Autodesk Inventor part; units mm, degrees
ref_plane "YZ Plane" through (0, 0, 0) normal (1, 0, 0) x (0, 1, 0)
ref_plane "XZ Plane" through (0, 0, 0) normal (0, 1, 0) x (-1, 0, 0)
ref_plane "XY Plane" through (0, 0, 0) normal (0, 0, 1) x (1, 0, 0)
ref_plane "Work Plane1" through (0, 0, 0) normal (0, 0, 1) x (1, 0, 0)
sketch "Sketch1" plane through (0, 0, 0) normal (0, 0, 1) x (1, 0, 0)
  line L0 (96.063, 0.903) -> (102.063, 0.903)
  line L1 (102.063, 0.903) -> (102.063, 3.903)
  line L2 (102.063, 3.903) -> (96.063, 3.903)
  line L3 (96.063, 3.903) -> (96.063, 0.903)
  line L4 (96.063, 0.903) -> (102.063, 3.903) construction
  line L5 (102.063, 0.903) -> (96.063, 3.903) construction
  line L6 (117.163, 0.353) -> (117.163, 4.453)
  line L7 (123.363, 4.453) -> (123.363, 0.353)
  line L8 (117.163, 2.403) -> (123.363, 2.403)
  line L9 (117.263, 3.903) -> (123.263, 3.903)
  line L10 (123.263, 3.903) -> (123.263, 0.903)
  line L11 (123.263, 0.903) -> (117.263, 0.903)
  line L12 (117.263, 0.903) -> (117.263, 3.903)
  line L13 (117.263, 3.903) -> (123.263, 0.903) construction
  line L14 (123.263, 3.903) -> (117.263, 0.903) construction
  point P0 (0, 0)
  point P1 (99.063, 2.403)
  point P2 (120.263, 2.403)
  dimension "d0" = 6
  dimension "d1" = 3
  dimension "d2" = 6
  dimension "d3" = 3
extrude "Extrusion1" add sketch "Sketch1" against normal blind 3
sketch "Sketch2" plane through (0, 0, 0) normal (0, 0, 1) x (1, 0, 0)
  line L0 (96.063, 0.903) -> (102.063, 0.903)
  line L1 (102.063, 0.903) -> (102.063, 3.903)
  line L2 (102.063, 3.903) -> (96.063, 3.903)
  line L3 (96.063, 3.903) -> (96.063, 0.903)
  line L4 (117.263, 3.903) -> (123.263, 3.903)
  line L5 (117.263, 0.903) -> (117.263, 3.903)
  line L6 (123.263, 0.903) -> (117.263, 0.903)
  line L7 (123.263, 3.903) -> (123.263, 0.903)
  point P0 (0, 0)
sketch "Sketch3" plane through (0, 0, 0) normal (0, 0, 1) x (1, 0, 0)
  line L0 (89.663, 3.903) -> (129.663, 3.903)
  line L1 (129.663, 3.903) -> (129.663, 0.903)
  line L2 (129.663, 0.903) -> (89.663, 0.903)
  line L3 (89.663, 0.903) -> (89.663, 3.903)
  line L4 (89.663, 3.903) -> (129.663, 0.903) construction
  line L5 (129.663, 3.903) -> (89.663, 0.903) construction
  point P0 (0, 0)
  point P1 (109.663, 2.403)
  dimension "d6" = 40
  dimension "d7" = 3
extrude "Extrusion2" add sketch "Sketch3" along normal blind 60
sketch "Sketch4" plane through (96.063, 3.903, -3) normal (0, 1, 0) x (1, 0, 0)
  line L0 (-6.4, -63) -> (33.6, -63)
  line L1 (33.6, -3) -> (33.6, -63)
  line L2 (-6.4, -63) -> (33.6, -63)
  line L3 (33.6, -63) -> (33.6, -23)
  line L4 (33.6, -23) -> (-6.4, -23)
  line L5 (-6.4, -23) -> (-6.4, -63)
  circle A0 centre (13.6, -43) radius 19
  line L6 (13.6, -43) -> (13.6, -27)
  line L7 (13.6, -27) -> (-2.4, -27)
  circle A1 centre (-2.4, -27) radius 1.6
  circle A2 centre (29.6, -27) radius 1.6
  line L8 (13.6, -43) -> (17.3038, -43)
  circle A3 centre (-2.4, -59) radius 1.6
  circle A4 centre (29.6, -59) radius 1.6
  point P0 (-96.063, -3)
  dimension "d10" = 40
  dimension "d11" = 38
  dimension "d12" = 16
  dimension "d13" = 16
  dimension "d14" = 3.2
extrude "Extrusion3" cut sketch "Sketch4" against normal through all contours A0 | A1 | A2 | A3 | A4
fillet "Fillet1" radius 2 2 edges at (89.663, 2.403, 60) (129.663, 2.403, 60)
sketch "Sketch5" plane through (117.263, 3.903, -3) normal (0, 1, 0) x (1, 0, 0)
  line L0 (-41.845, -71.0861) -> (34.1344, -71.0861)
  line L1 (34.1344, -71.0861) -> (34.1344, -32.9739)
  line L2 (34.1344, -32.9739) -> (-41.845, -32.9739)
  line L3 (-41.845, -32.9739) -> (-41.845, -71.0861)
  point P0 (-117.263, -3)
extrude "Extrusion4" cut sketch "Sketch5" against normal blind 40
fillet "Fillet2" radius 2 4 edges at (125.8023, 2.403, 29.9739) (93.5237, 2.403, 29.9739) (129.663, 2.403, 29.9739) (89.663, 2.403, 29.9739)
sketch "Sketch6" plane through (117.263, 3.903, -3) normal (0, 1, 0) x (1, 0, 0)
  line L0 (-9.2, 0) -> (-9.2, -3)
  line L1 (-6, 0) -> (-6, -3)
  line L2 (38.3326, -3) -> (-143.1956, -3)
  line L3 (0, -3) -> (-15.2, -3)
  line L4 (-7.6, -3) -> (-6.1, -3)
  line L5 (-6.1, -13.7) -> (-7.6, -13.7)
  line L6 (-7.6, -3) -> (-9.1, -3)
  line L7 (-9.1, -13.7) -> (-7.6, -13.7)
  line L8 (-9.1, -3) -> (-9.1, -9)
  line L9 (-9.1, -9) -> (-10.3, -9)
  line L10 (-10.3, -9) -> (-10.3, -11)
  line L11 (-10.3, -11) -> (-9.1, -11)
  line L12 (-9.1, -3) -> (-9.1, -9)
  line L13 (-9.1, -11) -> (-9.1, -13.7)
  line L14 (-7.6, -3) -> (-7.6, -5.4805)
  line L15 (-6.1, -3) -> (-6.1, -9)
  line L16 (-6.1, -9) -> (-4.9, -9)
  line L17 (-4.9, -9) -> (-4.9, -11)
  line L18 (-4.9, -11) -> (-6.1, -11)
  line L19 (-6.1, -11) -> (-6.1, -13.7)
  point P0 (-117.263, -3)
  dimension "d21" = 1.5
  dimension "d22" = 10.7
  dimension "d23" = 1.5
  dimension "d24" = 6
  dimension "d25" = 1.2
  dimension "d26" = 2
extrude "Extrusion5" cut sketch "Sketch6" against normal through all
sketch "Sketch7" plane through (0, 0, -3) normal (0, 0, -1) x (-1, 0, 0)
  point P0 (0, 0)
  point P1 (-109.663, 2.403)
properties part number "Fanmount_CPY1_CPY_CPY" material "Acetal Resin, Black"
Can you work these out from the model? Positions are in its coordinate system, mm. A direction names the side the tool comes from. Give positions to 0.01 mm unless a question says otherwise; leave off trailing zeros. Write each loop counter-clockwise with the first axis right and the second up, starting at its lowest first coordinate (ties: lowest second). Pieces come first, ordered by that corner, then holes. Notation, with made-up numbers: (17.5, 89) -> (64.5, 89) arc R28 ccw to (64.5, 111) -> close; hole circle Ø11 at (83, 83.5). An arc over 180 degrees is marked (long way). Write item = value, one per line.
(1) I need wall thicknesses on probe 1 along X at (y, z) = (1.8, 4.5); probe 2 along X at (y, z) = (3.05, 24); probe 3 along X at (y, z) = (3.35, 23). Which ranges of each line are inside material? Lowest first, please. Write a range as from..to.
Worked out:
probe_1 = 89.66..108.16, 111.16..129.66
probe_2 = 89.66..92.06, 95.26..99.42, 119.91..124.06, 127.26..129.66
probe_3 = 89.66..92.41, 94.91..101.18, 118.15..124.41, 126.91..129.66
(2) Suppose I cut it at C-C on x = 93. Write out the boundary of the cut face in (y, z).
Worked out:
outline = (0.9, 0) -> (3.9, 0) -> (3.9, 22.54) -> (0.9, 22.54) -> close; (0.9, 25.46) -> (3.9, 25.46) -> (3.9, 29.9) -> (0.9, 29.9) -> close
(3) Suppose I cut it at B-B on y = 2.3. Count the separate pieces of the cut face and the enclosed holes in it, then the cut area to 3 significant figures.
Worked out:
separate_pieces = 1
enclosed_holes = 2
area = 975 mm^2
(4) For faces 1 (the face through (112.363, 2, 7)), 2 (the face through (129.663, 2, 14)), 3 (the face through (110, 2, 10.7)), which set-ups out of +Z, -Z, +X, -X, +Y, -Y let a thin tool reach every point of the face, with its end or its side?
Worked out:
face_1 = +Y, -Y
face_2 = +Z, -Z, +X, +Y, -Y
face_3 = -Z, +Y, -Y
(5) Thinking about a two-plate mould opening in X: for faces 4 (the face through (95.19, 2.42, 23.52)), 5 (the face through (93, 2, 0)), 6 (the face through (90.26, 2.38, 29.4)), 7 (the face through (123.263, 2, -1)), which applies, released by +X, released by -X, zero draft, split by the parting line, or undercut?
Worked out:
face_4 = undercut
face_5 = zero draft
face_6 = released by -X
face_7 = released by +X
(6) I'm going to push flat-ended pins straight in: P1, Ø1.5, axis at x = 92, y = 2, coming from the -Z side; P2, Ø1, axis at x = 112, y = 2.5, coming from the +Z side; P3, Ø4, axis at x = 101.5, z = 24.5, coming from the -Y side; P4, Ø1.5, axis at y = 2, z = -1.5, coming from the +X side. Where does each tip first touch, or does it pass through?
Worked out:
P1 = 0
P2 = 21.21
P3 = 0.9
P4 = 123.26
(7) Suppose I cut it at D-D on z = 24. Write out the boundary of the cut face in (x, y), then the cut area to 3 significant figures.
Worked out:
outline = (89.66, 0.9) -> (92.06, 0.9) -> (92.06, 3.9) -> (89.66, 3.9) -> close; (95.26, 0.9) -> (99.42, 0.9) -> (99.42, 3.9) -> (95.26, 3.9) -> close; (119.91, 0.9) -> (124.06, 0.9) -> (124.06, 3.9) -> (119.91, 3.9) -> close; (127.26, 0.9) -> (129.66, 0.9) -> (129.66, 3.9) -> (127.26, 3.9) -> close
area = 39.3 mm^2
(8) Suppose I cut it at A-A on z = 2.5. Write out the boundary of the cut face in (x, y), then the cut area to 3 significant figures.
Worked out:
outline = (89.66, 0.9) -> (108.16, 0.9) -> (108.16, 3.9) -> (89.66, 3.9) -> close; (111.16, 0.9) -> (129.66, 0.9) -> (129.66, 3.9) -> (111.16, 3.9) -> close
area = 111 mm^2
